Work out the finished part from the listing and answer in its coordinate system (mm). Give positions to 0.01 mm unless a question says otherwise; leave off trailing zeros. Write each loop counter-clockwise with the first axis right and the second up, starting at its lowest first coordinate (ties: lowest second). Pieces come first, ordered by that corner, then holes.
1) Straight lines are drawn through the part: probe 1 along X at (y, z) = (-4.45, 239); probe 2 along X at (y, z) = (-0.95, 130.5); probe 3 along Z at (x, y) = (31.5, -0.25). For each, find the intervals that lie inside material, in ascending order.
2) Find section B-B (x = 151). Determine the outline of the cut face in (y, z), plus the area to 3 significant figures.
3) Find section C-C (y = -5.1). Determine the outline of the cut face in (x, z), plus the area to 3 significant figures.
4) Given pin 1 Ø0.9 at (y, z) = (-1.5, 79) entering from +X; pin 2 Ø1.5 at (x, y) = (113.5, -3) entering from -Z; pin 3 Ø0.9 at (y, z) = (-2, 68) entering from -X, each flat-ended and moving along its own axis, determine where each tip first touches the part or whether it passes through.
5) Find section A-A (z = 100.5). Determine the outline of the cut face in (x, y), plus the area to 3 significant figures.
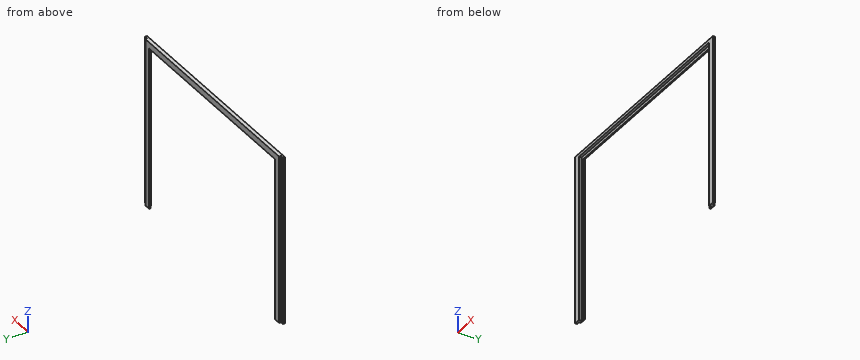
```python
from build123d import *

# Parameters (mm, degrees)
F1_DEPTH = 6
F2_W     = 330
F2_H     = 265
F3_DEPTH = 4
F4_W     = 3
F4_H     = 270
F5_DEPTH = 5
F6_W     = 3
F6_H     = 270
F7_DEPTH = 5


with BuildPart() as f1:
    # F0 (on Front) → F1 (new body)
    with BuildSketch(Plane.XZ):
        Polygon((0, 270), (0, 0), (10, 0), (10, 260), (330, 260), (330, 0), (340, 0), (340, 270), align=None)
    extrude(amount=F1_DEPTH)

    # F2 (on face) → F3 (cut)
    with BuildSketch(Plane.XZ.offset(6)):
        with Locations((170, 132.5)):
            Rectangle(F2_W, F2_H)
    extrude(amount=-F3_DEPTH, mode=Mode.SUBTRACT)

    # F4 (on face) → F5 (join)
    with BuildSketch(Plane(origin=(0, 0, 0), x_dir=(0, -1, 0), z_dir=(-1, 0, 0))):
        with Locations((4.5, 135)):
            Rectangle(F4_W, F4_H)
    extrude(amount=F5_DEPTH)

    # F6 (on face) → F7 (join)
    with BuildSketch(Plane.YZ.offset(340)):
        with Locations((-4.5, 135)):
            Rectangle(F6_W, F6_H)
    extrude(amount=F7_DEPTH)


solid = f1.part
```
Results:
1. probe 1: x = -5 to 5, 335 to 345
1. probe 2: x = 0 to 10, 330 to 340
1. probe 3: z = 260 to 270
2. outline: (-6, 265) - (-2, 265) - (-2, 260) - (0, 260) - (0, 270) - (-6, 270) - close
2. area: 40.0 mm2
3. outline: (-5, 0) - (5, 0) - (5, 265) - (335, 265) - (335, 0) - (345, 0) - (345, 270) - (-5, 270) - close
3. area: 7,050 mm2
4. pin 1: stops at x = 340
4. pin 2: stops at z = 265
4. pin 3: stops at x = 0
5. outline: (-5, -6) - (5, -6) - (5, -2) - (10, -2) - (10, 0) - (0, 0) - (0, -3) - (-5, -3) - close; (330, -2) - (335, -2) - (335, -6) - (345, -6) - (345, -3) - (340, -3) - (340, 0) - (330, 0) - close
5. area: 110 mm2
